from build123d import *

# Parameters (mm, degrees)
BOSS_EXTRUDE1_DEPTH = 5
SKETCH4_R           = 2
CUT_EXTRUDE1_DEPTH  = 10


with BuildPart() as part:
    # Sketch2 → Boss-Extrude1 (new body)
    with BuildSketch(Plane.XY):
        with BuildLine():
            Line((6.578363356, -21.516857009), (32.24208854, -37.05304733))
            Line((32.24208854, -37.05304733), (47.778278861, -11.389322146))
            Line((47.778278861, -11.389322146), (22.114553677, 4.146868175))
            ThreePointArc((22.114553677, 4.146868175), (0, 22.5), (-22.114553677, 4.146868175))
            Line((-22.114553677, 4.146868175), (-47.778278861, -11.389322146))
            Line((-47.778278861, -11.389322146), (-32.24208854, -37.05304733))
            Line((-32.24208854, -37.05304733), (-6.578363356, -21.516857009))
            ThreePointArc((-6.578363356, -21.516857009), (0, -22.5), (6.578363356, -21.516857009))
        make_face()
    extrude(amount=BOSS_EXTRUDE1_DEPTH)

    # Sketch4 → Cut-Extrude1 (cut)
    with BuildSketch(Plane.XY.offset(5)):
        with Locations((-40.911626277, -13.077244623)):
            Circle(SKETCH4_R)
        with Locations((-23.802476154, -2.719784409)):
            Circle(SKETCH4_R)
        with Locations((-13.44501594, -19.828934532)):
            Circle(SKETCH4_R)
        with Locations((-30.554166063, -30.186394746)):
            Circle(SKETCH4_R)
        with Locations((23.802476154, -2.719784409)):
            Circle(SKETCH4_R)
        with Locations((13.44501594, -19.828934532)):
            Circle(SKETCH4_R)
        with Locations((40.911626277, -13.077244623)):
            Circle(SKETCH4_R)
        with Locations((30.554166063, -30.186394746)):
            Circle(SKETCH4_R)
    extrude(amount=-CUT_EXTRUDE1_DEPTH, mode=Mode.SUBTRACT)


solid = part.part
The listing builds one solid part. Answer for the finished solid, in the listing's coordinates (mm). A direction names the side the tool comes from. Give positions to 0.01 mm unless a question says otherwise; leave off trailing zeros. Order: outer loops, then holes, each group sorted by start corner. A loop starts at its lowest first (then second) coordinate and runs counter-clockwise, first axis right, second up. Notation, with made-up numbers: (-34, -15) - (7, -15) arc R31 ccw to (7, 15) - close; hole circle Ø9 at (-18.75, 50). An arc over 180 degrees is marked (long way). Use one line per item in the form item = value.
1) Find section D-D on x = -7.5. Determine the outline of the cut face in (y, z).
Verdict:
outline = (-22.07, 0) - (21.21, 0) - (21.21, 5) - (-22.07, 5) - close
2) Consider probe 1 along X at (y, z) = (-4, 2.8); probe 2 along X at (y, z) = (-18.5, 2.4); probe 3 along Y at (x, z) = (0.5, 2.9). Determine where each line is inside the solid, lowest interval first. Write a range as [from, to].
Verdict:
probe_1 = [-35.57, -25.34], [-22.27, 22.27], [25.34, 35.57]
probe_2 = [-43.47, -14.94], [-11.95, 11.95], [14.94, 43.47]
probe_3 = [-22.49, 22.49]
3) Find section B-B on z = 3.5. Give the number of separate pieces and of enclosed holes in the cut face, and give its area (3 significant figures).
Verdict:
separate_pieces = 1
enclosed_holes = 8
area = 3,050 mm^2
4) Find section A-A on x = -41. Determine the outline of the cut face in (y, z), and give its area (3 significant figures).
Verdict:
outline = (-22.59, 0) - (-15.08, 0) - (-15.08, 5) - (-22.59, 5) - close; (-11.08, 0) - (-7.29, 0) - (-7.29, 5) - (-11.08, 5) - close
area = 56.5 mm^2
5) The mould has two halves that part along X. Classify faces 3 (the cylindrical face through (-11.537, -19.228, 2.535)), 4 (the cylindrical face through (0.436, 22.496, 2.465)), 5 (the flat face through (-40.12, -24.04, 2.46)): released by +X, released by -X, zero draft, split by the parting line, or undercut.
Verdict:
face_3 = undercut
face_4 = split by the parting line
face_5 = released by -X
6) For faces 1 (the flat face through (19.231, -29.176, 2.465)), 2 (the flat face through (39.9, -24.4, 2.5)), determine the directions among +Z, -Z, +X, -X, +Y, -Y from which every point of the face is accessible in a straight line to the end or side of a thin tool.
Verdict:
face_1 = +Z, -Z, -Y
face_2 = +Z, -Z, +X, -Y
7) Find section C-C on y = -23.5. Determine the outline of the cut face in (x, z), and give its area (3 significant figures).
Verdict:
outline = (-40.45, 0) - (-9.85, 0) - (-9.85, 5) - (-40.45, 5) - close; (9.85, 0) - (40.45, 0) - (40.45, 5) - (9.85, 5) - close
area = 306 mm^2
8) Each of these flat-tipped pins is pushed along its axis until it touches: pin 1 (3 mm diameter, centred on x = 40.91, y = -13.08, fed in from +Z); pin 2 (1.5 mm diameter, centred on x = 5.5, z = 1.5, fed in from -Y); pin 3 (3 mm diameter, centred on x = 37, z = 1.5, fed in from -Y); pin 4 (2 mm diameter, centred on y = -16.5, z = 1, fed in from -X). Where does it stop, or does it pass through?
Verdict:
pin_1 = through
pin_2 = -21.99
pin_3 = -31.67
pin_4 = -45.29
